Read the model definition and answer for the solid it produces. Units are mm, in the model's axes. A direction names the side the tool comes from. Coordinates: 2 decimals unless noted, no trailing zeros. Order: outer loops, then holes, each group sorted by start corner. A loop starts at its lowest first (then second) coordinate and runs counter-clockwise, first axis right, second up. Notation, with made-up numbers: (-12, -4) -> (2, -4) arc R10 ccw to (2, 11) -> close; hole circle Ø10 at (74, -10). An arc over 180 degrees is marked (long way). Use CSV: the item, a comma, the result in double quotes.
```python
from build123d import *

# Parameters (mm, degrees)
BOSS_EXTRUDE1_DEPTH = 32
FILLET1_R           = 7
CUT_EXTRUDE1_DEPTH  = 32
CUT_EXTRUDE2_DEPTH  = 32
CUT_EXTRUDE3_DEPTH  = 32
SKETCH7_R           = 3
BOSS_EXTRUDE2_DEPTH = 12
BOSS_EXTRUDE3_DEPTH = 4
SKETCH9_W           = 3
SKETCH9_H           = 2
SKETCH9_W_2         = 2
SKETCH9_H_2         = 3
CUT_EXTRUDE4_DEPTH  = 4
SKETCH10_R          = 7.5
BOSS_EXTRUDE4_DEPTH = 2
BOSS_EXTRUDE5_DEPTH = 2
BOSS_EXTRUDE6_DEPTH = 9
SKETCH17_R          = 4.5
CUT_EXTRUDE5_DEPTH  = 10


with BuildPart() as part:
    # Sketch1 → Boss-Extrude1 (new body)
    with BuildSketch(Plane(origin=(0, 0, 0), x_dir=(1, 0, 0), z_dir=(0, 1, 0))):
        Polygon((0, 0), (28, 0), (43, -10), (276, -10), (276, -5), (44.513878189, -5), (29.513878189, 5), (0, 5), align=None)
    extrude(amount=BOSS_EXTRUDE1_DEPTH)

    # Fillet1
    fillet1_edges = [part.edges().sort_by_distance(p)[0] for p in [
        (29.513878189, 16, -5),
        (44.513878189, 16, 5),
        (43, 16, 10),
        (28, 16, 0),
    ]]
    fillet(fillet1_edges, radius=FILLET1_R)

    # Sketch4 → Cut-Extrude1 (cut)
    with BuildSketch(Plane(origin=(0, 0, -5), x_dir=(-1, 0, 0), z_dir=(0, 0, -1))):
        with BuildLine():
            Line((-11, 32), (12.683379318, 39.348401976))
            Line((12.683379318, 39.348401976), (11.560507562, -17.356621714))
            Line((11.560507562, -17.356621714), (-11, 0))
            ThreePointArc((-11, 0), (0, 16), (-11, 32))
        make_face()
    extrude(amount=-CUT_EXTRUDE1_DEPTH, mode=Mode.SUBTRACT)

    # Sketch5 → Cut-Extrude2 (cut)
    with BuildSketch(Plane(origin=(0, 0, -5), x_dir=(-1, 0, 0), z_dir=(0, 0, -1))):
        Polygon((-276, 25), (-27.394448725, 31.56693909), (-27.394448725, 32), (-276, 32), align=None)
        Polygon((-27.394448725, 0), (-27.394448725, 0.43306091), (-276, 7), (-276, 0), align=None)
    extrude(amount=-CUT_EXTRUDE2_DEPTH, mode=Mode.SUBTRACT)

    # Sketch6 → Cut-Extrude3 (cut)
    with BuildSketch(Plane(origin=(0, 0, 5), x_dir=(-1, 0, 0), z_dir=(0, 0, -1))):
        with BuildLine():
            ThreePointArc((-276, 16.000000308), (-274.6681814, 21.205641364), (-271, 25.132075472))
            Line((-271, 25.132075472), (-276, 25))
            Line((-276, 25), (-276, 16.000000308))
        make_face()
        with BuildLine():
            ThreePointArc((-271, 6.867924528), (-274.668181548, 10.794358906), (-276, 16.000000308))
            Line((-276, 16.000000308), (-276, 7))
            Line((-276, 7), (-271, 6.867924528))
        make_face()
    extrude(amount=-CUT_EXTRUDE3_DEPTH, mode=Mode.SUBTRACT)

    # Sketch7 → Boss-Extrude2 (add)
    with BuildSketch(Plane.XY.offset(10)):
        with Locations((265.160519758, 16)):
            Circle(SKETCH7_R)
    extrude(amount=BOSS_EXTRUDE2_DEPTH)

    # Sketch8 → Boss-Extrude3 (add)
    with BuildSketch(Plane.XY.offset(22)):
        Polygon((270.93402245, 16), (268.047271104, 21), (262.273768412, 21), (259.387017066, 16), (262.273768412, 11), (268.047271104, 11), align=None)
    extrude(amount=BOSS_EXTRUDE3_DEPTH)

    # Sketch9 → Cut-Extrude4 (cut)
    with BuildSketch(Plane.XY.offset(26)):
        with Locations((267.660519758, 16)):
            Rectangle(SKETCH9_W, SKETCH9_H)
        with Locations((265.160519758, 18.5)):
            Rectangle(SKETCH9_W_2, SKETCH9_H_2)
        with Locations((265.160519758, 16)):
            Rectangle(SKETCH9_W_2, SKETCH9_H)
        with Locations((262.660519758, 16)):
            Rectangle(SKETCH9_W, SKETCH9_H)
        with Locations((265.160519758, 13.5)):
            Rectangle(SKETCH9_W_2, SKETCH9_H_2)
    extrude(amount=-CUT_EXTRUDE4_DEPTH, mode=Mode.SUBTRACT)

    # Sketch10 → Boss-Extrude4 (add)
    with BuildSketch(Plane.XY.offset(10)):
        with Locations((265.160519758, 16)):
            Circle(SKETCH10_R)
    extrude(amount=BOSS_EXTRUDE4_DEPTH)

    # Sketch11 → Boss-Extrude5 (add)
    with BuildSketch(Plane.XY):
        Polygon((27.528668482, 16), (22.332516059, 25), (11.940211214, 25), (6.744058791, 16), (11.940211214, 7), (22.332516059, 7), align=None)
    extrude(amount=BOSS_EXTRUDE5_DEPTH)

    # Sketch12 → Boss-Extrude6 (add)
    with BuildSketch(Plane.XY.offset(2)):
        Polygon((22.332516059, 7), (27.528668482, 16), (22.332516059, 25), (11.940211214, 25), (6.744058791, 16), (11.940211214, 7), align=None)
    extrude(amount=-BOSS_EXTRUDE6_DEPTH)

    # Sketch17 → Cut-Extrude5 (cut)
    with BuildSketch(Plane.XY.offset(2)):
        with Locations((17.136363636, 16)):
            Circle(SKETCH17_R)
    extrude(amount=-CUT_EXTRUDE5_DEPTH, mode=Mode.SUBTRACT)


solid = part.part
```
Item 1: Each of these flat-tipped pins is pushed along its axis until it touches: P1, Ø3, axis at x = 200.5, y = 3, coming from the +Z side; P2, Ø1.6, axis at y = 16, z = 24.5, coming from the -X side; P3, Ø13, axis at x = 17.5, y = 23.5, coming from the +Z side; P4, Ø1.5, axis at x = 263, z = 23, coming from the +Y side. Where does it stop, or does it pass through?
Return value:
P1,"passes through"
P2,"stops at x = 259.39"
P3,"stops at z = 2"
P4,"stops at y = 21"
Item 2: Straight lines are drawn through the part: line 1 along Z through (x, y) = (237.5, 9.5); line 2 along Z through (x, y) = (12, 9.5); line 3 along X through (y, z) = (24, 8.5). For each, find the intervals that lie inside material, in ascending order.
Return value:
line 1,"z = 5 to 10"
line 2,"z = -7 to 2"
line 3,"x = 40.75 to 272.47"
Item 3: The mould has two halves that part along Z. Classify faces 5 (the flat face through (35.42, 15.783, 4.946)), 6 (the flat face through (9.4, 20.6, 1)), 7 (the flat face through (19.3, 20.13, -7)), 8 (the flat face through (268, 18, 22)): +Z half, -Z half, draft (parallel to the pull), parting line (faces both ways), or undercut.
Return value:
face 5,"+Z half"
face 6,"draft"
face 7,"-Z half"
face 8,"undercut"
Item 4: A tool of negligible diameter and unlimited length cuts with its end or side. For faces 1 (the flat face through (19.3, 20.13, 2)), 2 (the flat face through (24.894, 11.437, -5.985)), 3 (the cylindrical face through (257.668, 16.33, 10.986)), 4 (the flat face through (9.306, 11.563, 0.986)), from which of +Z, -Z, +X, -X, +Y, -Y can it reach the whole face along a straight path? Write none if from no direction.
Return value:
face 1,"+Z, -X, +Y, -Y"
face 2,"-Z, +X, -Y"
face 3,"+Z"
face 4,"+Z, -X, -Y"
Item 5: Find section B-B, the plane x = 57.5. Give the vertices of the cut face in (y, z).
Return value:
outline,"(1.23, 5) -> (30.77, 5) -> (30.77, 10) -> (1.23, 10) -> close"
Item 6: Find section A-A, the plane x = 124. Give the vertices of the cut face in (y, z).
Return value:
outline,"(2.98, 5) -> (29.02, 5) -> (29.02, 10) -> (2.98, 10) -> close"
